from build123d import *

# Parameters (mm, degrees)
F1_DEPTH = 50.8
F2_R     = 5.08
F3_T     = -2.54


# Not quite as in the source:
# - a shell that OpenCascade refuses in one call is made with other operations: the cavity is built on its own and cut out


with BuildPart() as f1:
    # F0 (on Front) → F1 (new body)
    with BuildSketch(Plane.XZ):
        Polygon((-36.388931796, -2.8822999448), (2.8822999448, -36.388931796), (36.388931796, 2.8822999448), (-2.8822999448, 36.388931796), align=None)
    extrude(amount=F1_DEPTH)

    # F2
    f2_edges = [f1.edges().sort_by_distance(p)[0] for p in [
        (36.388932, -25.4, 2.8823),
        (-2.8823, -25.4, 36.388932),
        (16.753316, 0, 19.635616),
        (16.753316, -50.8, 19.635616),
        (-19.635616, -50.8, 16.753316),
        (-16.753316, -50.8, -19.635616),
        (19.635616, -50.8, -16.753316),
        (2.8823, -25.4, -36.388932),
        (19.635616, 0, -16.753316),
        (-36.388932, -25.4, -2.8823),
        (-16.753316, 0, -19.635616),
    ]]
    fillet(f2_edges, radius=F2_R)

    # F3: a shell. OpenCascade refuses it in one call, so the cavity is built on its own and cut out:
    # the body offset inwards by the wall thickness, plus a prism from it out through each open face.
    f3_core = offset(f1.part, amount=F3_T, mode=Mode.PRIVATE)
    f3_exits = [f3_core.faces().sort_by_distance(p)[0] for p in [
        (0, -48.26, 0),
    ]]
    add(f3_core, mode=Mode.SUBTRACT)
    extrude(f3_exits, amount=-F3_T, mode=Mode.SUBTRACT)


solid = f1.part
Check sheet for the modelled part. Datum: model origin and axes. Units: mm. A direction names the side the tool comes from. Round coordinates to 2 decimals unless told otherwise and drop trailing zeros. Order: outer loops, then holes, each group sorted by start corner. A loop starts at its lowest first (then second) coordinate and runs counter-clockwise, first axis right, second up.
(1) Cross-section at B-B, the plane y = -10.5. Enter the section's corners in (x, z), and give its area (3 significant figures).
(2) Access from +Z, -Z, +X, -X, +Y, -Y to the whole of each face (thin tool, end or side, straight path). Record for faces 4 (the flat face through (-15.33, -25.12, -17.51)), 5 (the flat face through (-15.58, -49.51, 13.68)), 6 (the cylindrical face through (-17.5, -1.53, -17.1)).
(3) Go/stop test with flat-tipped pins: P1, Ø6, axis at x = 12.5, y = -30, coming from the +Z side; P2, Ø5, axis at y = -9.5, z = 19.5, coming from the +X side; P3, Ø5, axis at x = -17.5, y = -18.5, coming from the +Z side. Record where each tip stops, or that it passes through.
(4) Scan lines: probe 1 along Y at (x, z) = (-13, 13.5); probe 2 along Z at (x, y) = (-19, -39); probe 3 along X at (y, z) = (-19, -12). Record each from-to range of solid material in increasing order.
(5) Draft check along X on faces 1 (the cylindrical face through (-2.66, -23.18, 34.295)), 2 (the cylindrical face through (-17.34, -47.5, 14.41)), 3 (the cylindrical face through (-18.722, -49.272, 15.592)). Enter one of: pulls with the +X half, pulls with the -X half, needs draft (parallel to the pull), parting line crosses it, or undercut.
(6) Cross-section at A-A, the plane y = -47. Enter the section's corners in (x, z), and give its area (3 significant figures).
Check sheet entries:
1. outline: (-33.09, 0.98) arc R5.08 ccw to (-32.52, -6.18) - (-0.98, -33.09) arc R5.08 ccw to (6.18, -32.52) - (33.09, -0.98) arc R5.08 ccw to (32.52, 6.18) - (0.98, 33.09) arc R5.08 ccw to (-6.18, 32.52) - close; hole (-31.16, -0.67) arc R2.54 ccw to (-30.88, -4.25) - (0.67, -31.16) arc R2.54 ccw to (4.25, -30.88) - (31.16, 0.67) arc R2.54 ccw to (30.88, 4.25) - (-0.67, 31.16) arc R2.54 ccw to (-4.25, 30.88) - close
1. area: 482 mm2
2. face 4: none
2. face 5: -Y
2. face 6: -Z, -X, +Y
3. P1: stops at z = 25.82
3. P2: stops at x = 19.84
3. P3: stops at z = 22.19
4. probe 1: y = -2.54 to 0
4. probe 2: z = -17.72 to -14.38, 13.58 to 17.5
4. probe 3: x = -25.7 to -21.79, 20.35 to 23.69
5. face 1: parting line crosses it
5. face 2: undercut
5. face 3: pulls with the -X half
6. outline: (-32.97, 0.88) arc R4.92 ccw to (-32.42, -6.05) - (-0.88, -32.97) arc R4.92 ccw to (6.05, -32.42) - (32.97, -0.88) arc R4.92 ccw to (32.42, 6.05) - (0.88, 32.97) arc R4.92 ccw to (-6.05, 32.42) - close; hole (-30.9, -0.89) arc R2.19 ccw to (-30.65, -3.98) - (0.89, -30.9) arc R2.19 ccw to (3.98, -30.65) - (30.9, 0.89) arc R2.19 ccw to (30.65, 3.98) - (-0.89, 30.9) arc R2.19 ccw to (-3.98, 30.65) - close
6. area: 512 mm2
